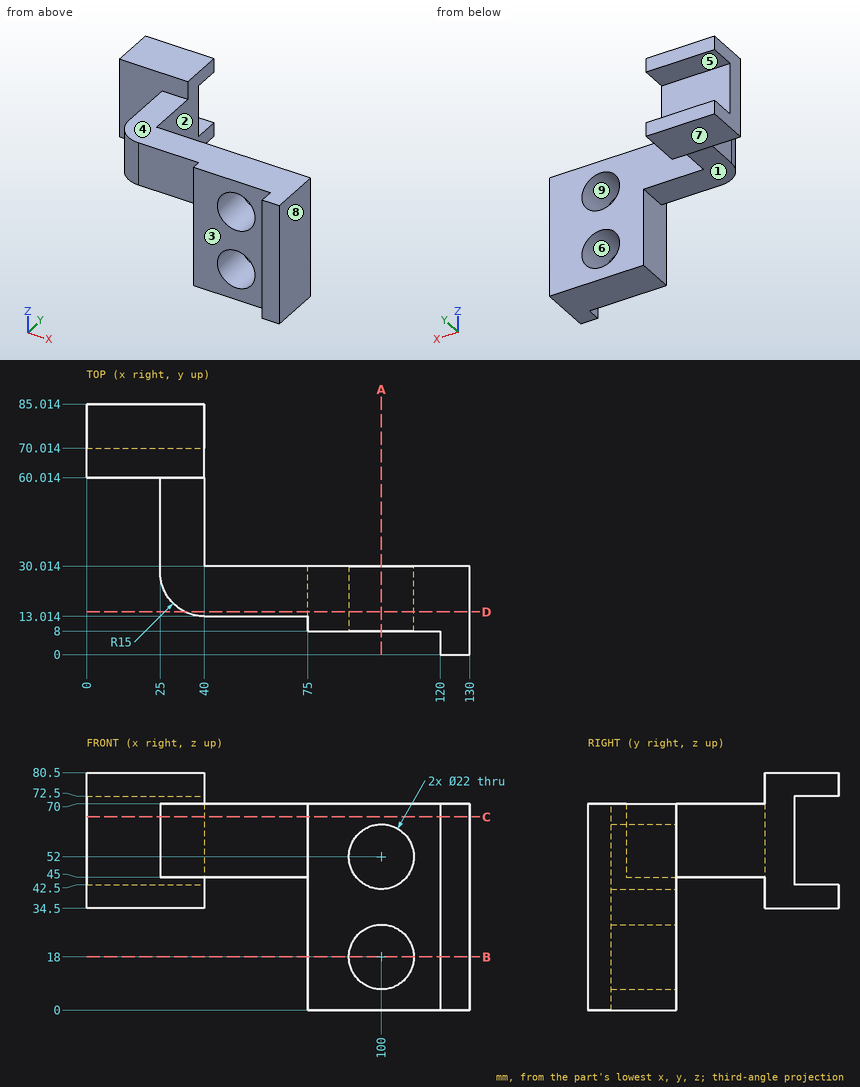
The figure shows three views and two pictorial views of one solid part (mm, origin at its lowest corner). Answer the questions. A direction names the side the tool comes from. Round coordinates to 2 decimals unless told otherwise and drop trailing zeros. Order: outer loops, then holes, each group sorted by start corner. A loop starts at its lowest first (then second) coordinate and runs counter-clockwise, first axis right, second up. Notation, with made-up numbers: (-4.5, 30.25) -> (40.5, 30.25) arc R25 cw to (40.5, 66.25) -> close; hole circle Ø1 at (12, 87). An arc over 180 degrees is marked (long way). Put each result on its own line as item: value.
Q1. Section B-B, the plane z = 18 is taken. Write down the section's boundary in (x, y) (1 decimal).
Results list:
outline: (75, 8) -> (89, 8) -> (89, 30) -> (75, 30) -> close; (111, 8) -> (120, 8) -> (120, 0) -> (130, 0) -> (130, 30) -> (111, 30) -> close
Q2. Which of the six approach directions +Z, -Z, +X, -X, +Y, -Y give full straight-line access (tool end or side, diameter ignored) to the marked faces 1, 2, 3, 4 and 5?
Results list:
face 1: -Z, -X, -Y
face 2: +Z, -Z, +X, +Y
face 3: +Z, -Z, -X, -Y
face 4: +Z, +X, -X, -Y
face 5: +X, -X, +Y
Q3. Determine the mould class of the marked faces 6, 7, 8 and 9 for opening direction X: pulls with the +X half, pulls with the -X half, needs draft (parallel to the pull), parting line crosses it, or undercut.
Results list:
face 6: undercut
face 7: needs draft
face 8: pulls with the +X half
face 9: undercut
Q4. Section A-A, the plane x = 100 is taken. Write down the section's boundary in (y, z) (1 decimal).
Results list:
outline: (8, 0) -> (30, 0) -> (30, 7) -> (8, 7) -> close; (8, 29) -> (30, 29) -> (30, 41) -> (8, 41) -> close; (8, 63) -> (30, 63) -> (30, 70) -> (8, 70) -> close
Q5. Section C-C, the plane z = 65.5 is taken. Write down the section's boundary in (x, y) (1 decimal).
Results list:
outline: (0, 60) -> (25, 60) -> (25, 28) arc R15 ccw to (40, 13) -> (75, 13) -> (75, 8) -> (120, 8) -> (120, 0) -> (130, 0) -> (130, 30) -> (40, 30) -> (40, 70) -> (0, 70) -> close
Q6. Each of these flat-tipped pins is pushed along its axis until it touches: P1, Ø8, axis at x = 93, y = 14, coming from the +Z side; P2, Ø7.5, axis at x = 52, z = 53, coming from the -Y side; P3, Ø22.5, axis at x = 103.5, z = 38.5, coming from the -Y side. Where does it stop, or does it pass through?
Results list:
P1: z = 70
P2: y = 13.01
P3: y = 8
Q7. Consider line 1 along Z through (x, y) = (100, 25); line 2 along Y through (x, z) = (70, 48.5) (1 decimal); line 3 along X through (y, z) = (47, 48.5). Determine where each line is inside the solid, lowest interval first.
Results list:
line 1: 0 to 7, 29 to 41, 63 to 70
line 2: 13 to 30
line 3: 25 to 40
Q8. Section D-D, the plane y = 14.5 is taken. Write down the section's boundary in (x, z), and give its area (3 significant figures).
Results list:
outline: (33.49, 45) -> (75, 45) -> (75, 0) -> (130, 0) -> (130, 70) -> (33.49, 70) -> close; hole circle Ø22 at (100, 18); hole circle Ø22 at (100, 52)
area: 4,130 mm^2
